Work out the finished part from the listing and answer in its coordinate system (mm). Face numbers are marked on the shaded views. A direction names the side the tool comes from. Coordinates: 2 decimals unless noted, no trailing zeros. Order: outer loops, then holes, each group sorted by start corner. A loop starts at its lowest first (then second) coordinate and runs counter-clockwise, first axis right, second up. Notation, with made-up numbers: (48, 65.5) -> (79, 65.5) arc R13 ccw to (79, 72.5) -> close; hole circle Ø7 at (-31, -32). An arc over 180 degrees is marked (long way). Use one line per item in the form item = value.
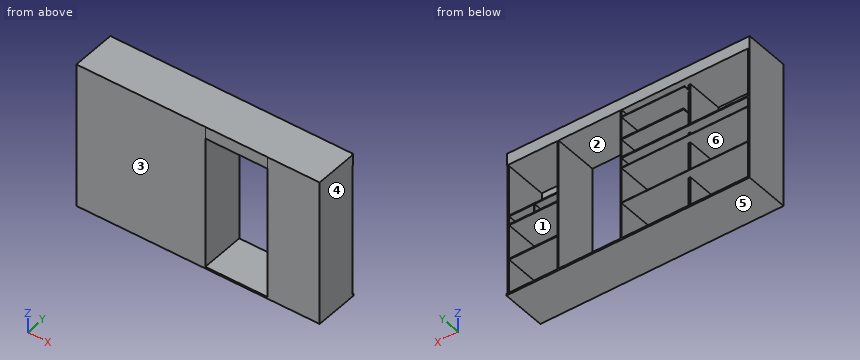
from build123d import *

# Parameters (mm, degrees)
F0_W      = 514.1673088074
F0_H      = 94.2290462554
F1_DEPTH  = 3.81
F2_W      = 2.2902190685
F2_H      = 94.2290462554
F3_DEPTH  = 304.8
F4_W      = 3.202021122
F4_H      = 90.812921524
F5_DEPTH  = 304.8
F6_W      = 1.6730939969
F6_H      = 94.2290462554
F7_DEPTH  = 304.8
F8_W      = 3.8608312607
F8_H      = 94.2290462554
F9_DEPTH  = 304.8
F10_W     = 3.5790838301
F10_H     = 78.3394947648
F11_DEPTH = 304.8
F12_W     = 272.5380798802
F12_H     = 308.61
F13_DEPTH = 0.254
F14_W     = 110.2488040924
F14_H     = 308.61
F15_DEPTH = 0.254
F16_W     = 90.558921524
F16_H     = 2.1528995848
F17_DEPTH = 105.41
F18_W     = 90.558921524
F18_H     = 2.4020688844
F19_DEPTH = 106.934
F20_W     = 90.558921524
F20_H     = 2.1886378527
F21_DEPTH = 106.934
F22_W     = 1.4953613281
F22_H     = 90.558921524
F23_DEPTH = 18.542
F24_R     = 2.7883656223
F25_DEPTH = 106.68
F26_W     = 93.9750462554
F26_H     = 1.1749916458
F27_DEPTH = 268.224
F28_W     = 93.9750462554
F28_H     = 2.5478154421
F29_DEPTH = 270.256
F30_W     = 93.9750462554
F30_H     = 1.2798203731
F31_DEPTH = 269.24
F32_W     = 93.9750462554
F32_H     = 1.3391077518
F33_DEPTH = 133.35
F34_W     = 93.9750462554
F34_H     = 2.4402439594
F35_DEPTH = 131.318
F36_R     = 1.6466720005
F37_DEPTH = 136.906
F38_W     = 512.9730403423
F38_H     = 93.9750462554
F39_DEPTH = 25.4


with BuildPart() as f1:
    # F0 (on Top) → F1 (new body)
    with BuildSketch(Plane.XY):
        with Locations((-2.9884278774, -84.9680285901)):
            Rectangle(F0_W, F0_H)
    extrude(amount=F1_DEPTH)

    # F2 (on face) → F3 (join)
    with BuildSketch(Plane.XY.offset(3.81)):
        with Locations((144.9915319681, -84.9680285901)):
            Rectangle(F2_W, F2_H)
    extrude(amount=F3_DEPTH)

    # F4 (on face) → F5 (join)
    with BuildSketch(Plane.XY.offset(3.81)):
        with Locations((252.4942159653, -86.6760909557)):
            Rectangle(F4_W, F4_H)
    extrude(amount=F5_DEPTH)

    # F6 (on face) → F7 (join)
    with BuildSketch(Plane.XY.offset(3.81)):
        with Locations((11.6294506006, -84.9680285901)):
            Rectangle(F6_W, F6_H)
    extrude(amount=F7_DEPTH)

    # F8 (on face) → F9 (join)
    with BuildSketch(Plane.XY.offset(3.81)):
        with Locations((-258.1416666508, -84.9680285901)):
            Rectangle(F8_W, F8_H)
    extrude(amount=F9_DEPTH)

    # F10 (on face) → F11 (join)
    with BuildSketch(Plane.XY.offset(3.81)):
        with Locations((-120.9196317941, -92.9128043354)):
            Rectangle(F10_W, F10_H)
    extrude(amount=F11_DEPTH)

    # F12 (on face) → F13 (join)
    with BuildSketch(Plane.XZ.offset(132.0825517178)):
        with Locations((-123.803042341, 154.305)):
            Rectangle(F12_W, F12_H)
    extrude(amount=-F13_DEPTH)

    # F14 (on face) → F15 (join)
    with BuildSketch(Plane.XZ.offset(132.0825517178)):
        with Locations((198.9708244801, 154.305)):
            Rectangle(F14_W, F14_H)
    extrude(amount=-F15_DEPTH)

    # F16 (on face) → F17 (join)
    with BuildSketch(Plane(origin=(250.8932054043, 0, 0), x_dir=(0, -1, 0), z_dir=(-1, 0, 0))):
        with Locations((86.5490909557, 155.1335502076)):
            Rectangle(F16_W, F16_H)
    extrude(amount=F17_DEPTH)

    # F18 (on face) → F19 (join)
    with BuildSketch(Plane(origin=(250.8932054043, 0, 0), x_dir=(0, -1, 0), z_dir=(-1, 0, 0))):
        with Locations((86.5490909557, 80.1345846498)):
            Rectangle(F18_W, F18_H)
    extrude(amount=F19_DEPTH)

    # F20 (on face) → F21 (join)
    with BuildSketch(Plane(origin=(250.8932054043, 0, 0), x_dir=(0, -1, 0), z_dir=(-1, 0, 0))):
        with Locations((86.5490909557, 174.4099780917)):
            Rectangle(F20_W, F20_H)
    extrude(amount=F21_DEPTH)

    # F22 (on face) → F23 (join)
    with BuildSketch(Plane.XY.offset(156.21)):
        with Locations((197.7672427893, -86.5490909557)):
            Rectangle(F22_W, F22_H)
    extrude(amount=F23_DEPTH)

    # F24 (on face) → F25 (join)
    with BuildSketch(Plane(origin=(250.8932054043, 0, 0), x_dir=(0, -1, 0), z_dir=(-1, 0, 0))):
        with Locations((86.5490909557, 288.2337272167)):
            Circle(F24_R)
    extrude(amount=F25_DEPTH)

    # F26 (on face) → F27 (join)
    with BuildSketch(Plane(origin=(10.7929036021, 0, 0), x_dir=(0, -1, 0), z_dir=(-1, 0, 0))):
        with Locations((84.8410285901, 156.7974958229)):
            Rectangle(F26_W, F26_H)
    extrude(amount=F27_DEPTH)

    # F28 (on face) → F29 (join)
    with BuildSketch(Plane(origin=(10.7929036021, 0, 0), x_dir=(0, -1, 0), z_dir=(-1, 0, 0))):
        with Locations((84.8410285901, 179.0851131082)):
            Rectangle(F28_W, F28_H)
    extrude(amount=F29_DEPTH)

    # F30 (on face) → F31 (join)
    with BuildSketch(Plane(origin=(10.7929036021, 0, 0), x_dir=(0, -1, 0), z_dir=(-1, 0, 0))):
        with Locations((84.8410285901, 80.6499101865)):
            Rectangle(F30_W, F30_H)
    extrude(amount=F31_DEPTH)

    # F32 (on face) → F33 (join)
    with BuildSketch(Plane(origin=(10.7929036021, 0, 0), x_dir=(0, -1, 0), z_dir=(-1, 0, 0))):
        with Locations((84.8410285901, 267.7811831236)):
            Rectangle(F32_W, F32_H)
    extrude(amount=F33_DEPTH)

    # F34 (on face) → F35 (join)
    with BuildSketch(Plane(origin=(10.7929036021, 0, 0), x_dir=(0, -1, 0), z_dir=(-1, 0, 0))):
        with Locations((84.8410285901, 219.618961215)):
            Rectangle(F34_W, F34_H)
    extrude(amount=F35_DEPTH)

    # F36 (on face) → F37 (join)
    with BuildSketch(Plane(origin=(-122.7091737092, 0, 0), x_dir=(0, -1, 0), z_dir=(-1, 0, 0))):
        with Locations((94.4481417537, 294.7028875351)):
            Circle(F36_R)
    extrude(amount=F37_DEPTH)

    # F38 (on face) → F39 (join)
    with BuildSketch(Plane.XY.offset(308.61)):
        with Locations((-3.5855621099, -84.8410285901)):
            Rectangle(F38_W, F38_H)
    extrude(amount=-F39_DEPTH)


solid = f1.part
(1) The mould has two halves that part along Z. Classify the marked faces 4, 5 and 6: released by +Z, released by -Z, zero draft, split by the parting line, or undercut.
Data:
face_4 = zero draft
face_5 = released by -Z
face_6 = undercut
(2) Section C-C on x = -39 is taken. Write down the section's boundary in (y, z) (1 decimal).
Data:
outline = (-132.1, 0) -> (-37.9, 0) -> (-37.9, 3.8) -> (-131.8, 3.8) -> (-131.8, 80) -> (-37.9, 80) -> (-37.9, 81.3) -> (-131.8, 81.3) -> (-131.8, 156.2) -> (-37.9, 156.2) -> (-37.9, 157.4) -> (-131.8, 157.4) -> (-131.8, 177.8) -> (-37.9, 177.8) -> (-37.9, 180.4) -> (-131.8, 180.4) -> (-131.8, 218.4) -> (-37.9, 218.4) -> (-37.9, 220.8) -> (-131.8, 220.8) -> (-131.8, 267.1) -> (-37.9, 267.1) -> (-37.9, 268.5) -> (-131.8, 268.5) -> (-131.8, 283.2) -> (-37.9, 283.2) -> (-37.9, 308.6) -> (-132.1, 308.6) -> close
(3) Section A-A on x = 136.5 is taken. Write down the section's boundary in (y, z), plus the area to 3 significant figures.
Data:
outline = (-132.08, 0) -> (-37.85, 0) -> (-37.85, 3.81) -> (-132.08, 3.81) -> close; (-131.83, 283.21) -> (-37.85, 283.21) -> (-37.85, 308.61) -> (-131.83, 308.61) -> close
area = 2,750 mm²
(4) Section D-D on z = 164 is taken. Write down the section's boundary in (x, y), plus the area to 3 significant figures.
Data:
outline = (-260.07, -132.08) -> (12.47, -132.08) -> (12.47, -37.85) -> (10.79, -37.85) -> (10.79, -131.83) -> (-119.13, -131.83) -> (-119.13, -53.74) -> (-122.71, -53.74) -> (-122.71, -131.83) -> (-256.21, -131.83) -> (-256.21, -37.85) -> (-260.07, -37.85) -> close; (143.85, -132.08) -> (254.1, -132.08) -> (254.1, -41.27) -> (250.89, -41.27) -> (250.89, -131.83) -> (198.51, -131.83) -> (198.51, -41.27) -> (197.02, -41.27) -> (197.02, -131.83) -> (146.14, -131.83) -> (146.14, -37.85) -> (143.85, -37.85) -> close
area = 1,540 mm²
(5) Section B-B on z = 129 is taken. Write down the section's boundary in (x, y).
Data:
outline = (-260.07, -132.08) -> (12.47, -132.08) -> (12.47, -37.85) -> (10.79, -37.85) -> (10.79, -131.83) -> (-119.13, -131.83) -> (-119.13, -53.74) -> (-122.71, -53.74) -> (-122.71, -131.83) -> (-256.21, -131.83) -> (-256.21, -37.85) -> (-260.07, -37.85) -> close; (143.85, -132.08) -> (254.1, -132.08) -> (254.1, -41.27) -> (250.89, -41.27) -> (250.89, -131.83) -> (146.14, -131.83) -> (146.14, -37.85) -> (143.85, -37.85) -> close
(6) Each of these flat-tipped pins is pushed along its axis until it touches: P1, Ø22.5, axis at x = -32.5, z = 102.5, coming from the +Y side; P2, Ø4, axis at x = -121, z = 130, coming from the +Y side. Where does it stop, or does it pass through?
Data:
P1 = -131.83
P2 = -53.74
(7) Straight lines are drawn through the part: line 1 along X through (y, z) = (-99, 224); line 2 along X through (y, z) = (-42, 262.5); line 3 along Z through (x, y) = (-159, -88.5) (3 decimals). For each, find the intervals that lie inside material, in ascending order.
Data:
line_1 = -260.07 to -256.21, -122.71 to -119.13, 10.79 to 12.47, 143.85 to 146.14, 250.89 to 254.1
line_2 = -260.07 to -256.21, 10.79 to 12.47, 143.85 to 146.14, 250.89 to 254.1
line_3 = 0 to 3.81, 80.01 to 81.29, 156.21 to 157.385, 177.811 to 180.359, 283.21 to 308.61
(8) Which of the six approach directions +Z, -Z, +X, -X, +Y, -Y give full straight-line access (tool end or side, diameter ignored) to the marked faces 1, 2 and 3?
Data:
face_1 = +Y
face_2 = +Y, -Y
face_3 = +Z, -Z, +X, -X, -Y
